```python
from build123d import *

# Parameters (mm, degrees)
F0_W        = 25.4
F0_H        = 254
F0_R        = 9.525
F1_DEPTH    = 25.4
F2_R        = 12.69999
F3_R        = 5.715
F4_DEPTH    = 26.67
F6_DEPTH    = 25.4
F7_T1_DEPTH = 69.85


# Not quite as in the source:
# - a fillet or chamfer that OpenCascade refuses, or shapes differently, is made with other operations: its cross-section is extruded or revolved along the edge and cut away or added
# - a fillet or chamfer is up to 0.001 mm smaller than in the source, because OpenCascade refuses the exact size


with BuildPart() as f1:
    # F0 (on Top) → F1 (new body)
    with BuildSketch(Plane.XY):
        with Locations((-33.2050182253, 13.4569510469)):
            Rectangle(F0_W, F0_H)
        with Locations((-33.2050182253, 124.5819510469)):
            Circle(F0_R, mode=Mode.SUBTRACT)
    extrude(amount=-F1_DEPTH)

    # F2 (radius 12.7 in the source; OpenCascade refuses exactly that, so slightly less here)
    f2_edges = [f1.edges().sort_by_distance(p)[0] for p in [
        (-45.905018, 140.456951, -12.7),
        (-20.505018, 140.456951, -12.7),
    ]]
    fillet(f2_edges, radius=F2_R)

    # F3 (on face) → F4 (cut)
    with BuildSketch(Plane.XZ.offset(113.5430489531)):
        with Locations((-33.2050182253, -6.2401448376)):
            Circle(F3_R)
    extrude(amount=-F4_DEPTH, mode=Mode.SUBTRACT)

    # F5 (on face) → F6 (cut)
    with BuildSketch(Plane(origin=(0, 0, -25.4), x_dir=(1, 0, 0), z_dir=(0, 0, -1))):
        with BuildLine():
            ThreePointArc((-33.2050182253, 81.7930489531), (-37.6951462858, 70.9529208925), (-26.8550182253, 75.4430489531))
            ThreePointArc((-26.8550182253, 75.4430489531), (-28.7148901648, 79.9331770136), (-33.2050182253, 81.7930489531))
        make_face()
    extrude(amount=-F6_DEPTH, mode=Mode.SUBTRACT)

    # F7: fillet of radius 8.89 on 1 edges, made by hand

    # F7_s2 → F7_t1 (cut)
    with BuildSketch(Plane.XY.offset(-47.625)):
        with BuildLine():
            ThreePointArc((-20.5050182253, -104.6530489531), (-23.1088389406, -110.9392282378), (-29.3950182253, -113.5430489531))
            Line((-29.3950182253, -113.5430489531), (-20.5050182253, -113.5430489531))
            Line((-20.5050182253, -113.5430489531), (-20.5050182253, -104.6530489531))
        make_face()
    extrude(amount=F7_T1_DEPTH, mode=Mode.SUBTRACT)


solid = f1.part
```
Verification items for the finished model (mm, model axes). A direction names the side the tool comes from. Coordinates: 2 decimals unless noted, no trailing zeros. Loops run counter-clockwise (first coordinate to the right, second up) from the corner with the lowest first, then second, coordinate; pieces in that order, holes last. Notation, with made-up numbers: (-8.75, 26) -> (3.25, 26) arc R16 cw to (3.25, 37) -> close; hole circle Ø10 at (-16.75, 83.5). An arc over 180 degrees is marked (long way). Answer in a Markdown table with one row per item. Add a question column.
1. Material ranges on probe 1 along Y at (x, z) = (-35, -5.25); probe 2 along Y at (x, z) = (-36.75, -6.25); probe 3 along Y at (x, z) = (-40.5, -17.5), recorded low to high. Write a range as [from, to].
2. Access from +Z, -Z, +X, -X, +Y, -Y to the whole of each face (thin tool, end or side, straight path). Record for faces 1 (the face through (-40, -113.543, -15)), 2 (the face through (-27.926, -100.395, -8.429)).
3. Draft check along X on faces 3 (the face through (-24.324, 136.835, -12.878)), 4 (the face through (-33, 15, 0)), 5 (the face through (-28.81, 116.13, -12.52)). Enter one of: +X half, -X half, draft (parallel to the pull), parting line (faces both ways), or undercut.
4. Section check A-A, the plane y = 120. Enter the section's corners in (x, z), then the cut area to 3 significant figures.
5. Depth check by flat-ended pin: P1, Ø1.5, axis at x = -26, z = -5.5, coming from the -Y side; P2, Ø5.5, axis at x = -34, z = -5.5, coming from the -Y side. Enter the tip coordinate at first touch or a pass-through.
6. Section check C-C, the plane z = -22. Give the number of separate pieces and of enclosed holes in the cut face, then the cut area to 3 significant figures.
7. Section check D-D, the plane y = -94.5. Enter the section's corners in (x, z) (3 decimals).
8. Section check B-B, the plane x = -36.5. Enter the section's corners in (y, z), then the cut area to 3 significant figures.
Derived:
| question | item | result |
|---|---|---|
| 1 | probe 1 | y = [-86.87, -81.53], [-69.35, 115.23], [133.94, 140.33] |
| 1 | probe 2 | y = [-86.87, -80.71], [-70.17, 115.74], [133.42, 139.95] |
| 1 | probe 3 | y = [-113.54, 118.46], [130.71, 138.15] |
| 2 | face 1 | +Z, -Z, +X, -X, -Y |
| 2 | face 2 | -Y |
| 3 | face 3 | +X half |
| 3 | face 4 | draft |
| 3 | face 5 | undercut |
| 4 | outline | (-45.91, -25.4) -> (-41.56, -25.4) -> (-41.56, 0) -> (-45.91, 0) -> close; (-24.85, -25.4) -> (-20.51, -25.4) -> (-20.51, 0) -> (-24.85, 0) -> close |
| 4 | area | 221 mm² |
| 5 | P1 | stops at y = -113.14 |
| 5 | P2 | stops at y = -86.87 |
| 6 | separate pieces | 1 |
| 6 | enclosed holes | 2 |
| 6 | area | 5,950 mm² |
| 7 | outline | (-45.905, -25.4) -> (-20.505, -25.4) -> (-20.505, 0) -> (-45.905, 0) -> close; hole circle Ø11.43 at (-33.205, -6.24) |
| 8 | outline | (-113.54, -25.4) -> (-80.87, -25.4) -> (-80.87, 0) -> (-113.54, 0) -> (-113.54, -1.57) -> (-86.87, -1.57) -> (-86.87, -10.91) -> (-113.54, -10.91) -> close; (-70.01, -25.4) -> (115.65, -25.4) -> (115.65, 0) -> (-70.01, 0) -> close; (133.52, -25.4) -> (140.02, -25.4) -> (140.02, 0) -> (133.52, 0) -> close |
| 8 | area | 5,460 mm² |
